Can you work these out from the model? Positions are in its coordinate system, mm. A direction names the side the tool comes from. Coordinates: 2 decimals unless noted, no trailing zeros. Write each loop counter-clockwise with the first axis right and the second up, starting at its lowest first coordinate (ties: lowest second). Pieces come first, ordered by that corner, then holes. Notation, with made-up numbers: (5.25, -40) -> (60.25, -40) arc R18 cw to (60.25, -23) -> close; hole circle Ø3 at (-28, -9). An arc over 180 degrees is marked (long way). Answer as CSV lines item,"result". Start each with the question number.
```python
from build123d import *

# Parameters (mm, degrees)
SKETCH1_R                    = 2.5
BASE_FLANGE1_DEPTH           = 3
EDGE_FLANGE1_STRIP_W         = 13.4732
EDGE_FLANGE1_STRIP_H         = 3
EDGE_FLANGE1_STRIP_CUT_DEPTH = 54
EDGE_FLANGE1_DEPTH           = 54
CUT_EXTRUDE1_START           = 16
CUT_EXTRUDE1_DEPTH           = 22
SKETCH10_R                   = 2.5
CUT_EXTRUDE2_DEPTH           = 10
SKETCH11_W                   = 22
SKETCH11_H                   = 16
SKETCH11_R                   = 2.5
BOSS_EXTRUDE1_DEPTH          = 3


# Read off the part's stored shape, not the designer's step: Cut-Extrude1
# Sheet-metal steps are written as plain solids
with BuildPart() as part:
    # Sketch1 → Base-Flange1 (new body)
    with BuildSketch(Plane(origin=(0, 0, 0), x_dir=(1, 0, 0), z_dir=(0, 1, 0))):
        with BuildLine():
            Line((0, 0), (54, 0))
            Line((54, 0), (54, 11))
            ThreePointArc((54, 11), (52.535533906, 14.535533906), (49, 16))
            Line((49, 16), (5, 16))
            ThreePointArc((5, 16), (1.464466094, 14.535533906), (0, 11))
            Line((0, 11), (0, 0))
        make_face()
        with Locations(Location((8, 8, 0), (0, 0, 270))):
            Circle(SKETCH1_R, mode=Mode.SUBTRACT)
        with Locations(Location((46, 8, 0), (0, 0, 90))):
            Circle(SKETCH1_R, mode=Mode.SUBTRACT)
    extrude(amount=-BASE_FLANGE1_DEPTH)

    # Edge-Flange1 strip (across the edge) → Edge-Flange1 strip cut (cut)
    with BuildSketch(Plane(origin=(0, 0, 0), x_dir=(0, 0, -1), z_dir=(1, 0, 0))):
        with Locations((-6, -1.5)):
            Rectangle(EDGE_FLANGE1_STRIP_W, EDGE_FLANGE1_STRIP_H)
    extrude(amount=EDGE_FLANGE1_STRIP_CUT_DEPTH, mode=Mode.SUBTRACT)

    # Edge-Flange1 section (across the edge) → Edge-Flange1 (add)
    with BuildSketch(Plane(origin=(0, 0, 0), x_dir=(0, 0, -1), z_dir=(1, 0, 0))):
        with BuildLine():
            Line((-3, 0.7366), (-3, 24))
            Line((-3, 24), (0, 24))
            Line((0, 24), (0, 0.7366))
            ThreePointArc((0, 0.7366), (0.215745145, 0.215745145), (0.7366, 0))
            Line((0.7366, 0), (0.7366, -3))
            ThreePointArc((0.7366, -3), (-1.905575199, -1.905575199), (-3, 0.7366))
        make_face()
    extrude(amount=EDGE_FLANGE1_DEPTH)

    # Cut-Extrude1 outline → Cut-Extrude1 (cut)
    with BuildSketch(Plane.YZ.offset(CUT_EXTRUDE1_START)):
        with BuildLine():
            Line((-2.926677222, 0), (0.014454199, -0.591393245))
            ThreePointArc((0.014454199, -0.591393245), (0.269898669, -0.166714548), (0.7366, 0))
            Line((0.7366, 0), (24, 0))
            Line((24, 0), (24, 3))
            Line((24, 3), (0.7366, 3))
            ThreePointArc((0.7366, 3), (-1.630867001, 2.154295979), (-2.926677222, 0))
        make_face()
    extrude(amount=CUT_EXTRUDE1_DEPTH, mode=Mode.SUBTRACT)

    # Sketch10 → Cut-Extrude2 (cut)
    with BuildSketch(Plane.XY.offset(3)):
        with BuildLine():
            ThreePointArc((46, 24), (51.656854249, 21.656854249), (54, 16))
            Line((54, 16), (54, 24))
            Line((54, 24), (46, 24))
        make_face()
        with Locations((46, 16)):
            Circle(SKETCH10_R)
        with Locations((8, 16)):
            Circle(SKETCH10_R)
        with BuildLine():
            ThreePointArc((0, 16), (2.343145751, 21.656854249), (8, 24))
            Line((8, 24), (0, 24))
            Line((0, 24), (0, 16))
        make_face()
    extrude(amount=-CUT_EXTRUDE2_DEPTH, mode=Mode.SUBTRACT)

    # Sketch11 → Boss-Extrude1 (add)
    with BuildSketch(Plane.XY.offset(3)):
        with Locations((27, 16)):
            Rectangle(SKETCH11_W, SKETCH11_H)
        with Locations((27, 16)):
            Circle(SKETCH11_R, mode=Mode.SUBTRACT)
    extrude(amount=-BOSS_EXTRUDE1_DEPTH)


solid = part.part
```
Q1. Which directions (+Z, -Z, +X, -X, +Y, -Y) give clear straight access to the entire face, cutting with the end or side of a thin tool? Please do faces 1 (the face through (53, -1, -14)), 2 (the face through (27, 13, 0)).
Q2. I need wall thicknesses on L1, parallel to X at y = -1.6, z = -8; L2, parallel to Y at x = 27, z = 2.2; L3, parallel to Z at x = 14.5, y = 3.75. Which ranges of each line are inside material? Lowest first, please.
Q3. Imagine slicing it at B-B (z = -8). Write out the boundary of the cut face in (x, y).
Q4. Imagine slicing it at C-C (z = -14). Write out the boundary of the cut face in (x, y), then the cut area to 3 significant figures.
Q5. For pin 1 (10 mm diameter, centred on x = 44, z = -2.5, fed in from +Y); pin 2 (0.9 mm diameter, centred on x = 26.5, z = 1.5, fed in from -Y); pin 3 (6 mm diameter, centred on x = 8, z = -8, fed in from +Y), each with a flat end and sliding along its axis, tell me the tip position at first contact or that it passes through.
Q6. If we mould it in two halves opening along X, with no side actions, what happens to faces 3 (the face through (54, 4, 1)), 4 (the face through (10.31, 15.04, 1.52)), 5 (the face through (16, 2, 1)), 6 (the face through (27, 0, -8))? For each: released by +X, released by -X, zero draft, split by the parting line, or undercut.
Q7. Imagine slicing it at A-A (x = 23). Write out the boundary of the cut face in (y, z), then the cut area to 3 significant figures.
Q8. Imagine slicing it at D-D (y = 10.5). Write out the boundary of the cut face in (x, z).
Entries:
1,face 1,"-Z, +X, +Y, -Y"
1,face 2,"-Z, +X, -X, +Y"
2,L1,"0 to 5.5, 10.5 to 43.5, 48.5 to 54"
2,L2,"8 to 13.5, 18.5 to 24"
2,L3,"0 to 3"
3,outline,"(0, -3) -> (5.5, -3) -> (5.5, 0) -> (0, 0) -> close; (10.5, -3) -> (43.5, -3) -> (43.5, 0) -> (10.5, 0) -> close; (48.5, -3) -> (54, -3) -> (54, 0) -> (48.5, 0) -> close"
4,outline,"(1, -3) -> (53, -3) -> (53, 0) -> (1, 0) -> close"
4,area,"156 mm2"
5,pin 1,"y = 24"
5,pin 2,"y = 8"
5,pin 3,"y = 0"
6,face 3,"released by +X"
6,face 4,"undercut"
6,face 5,"undercut"
6,face 6,"zero draft"
7,outline,"(-3, -16) -> (0, -16) -> (0, -0.74) arc R0.74 cw to (0.01, -0.59) -> (-2.93, 0) arc R3.74 ccw to (-3, -0.74) -> close; (8, 0) -> (24, 0) -> (24, 3) -> (8, 3) -> close"
7,area,"95.1 mm2"
8,outline,"(0, 0) -> (54, 0) -> (54, 3) -> (0, 3) -> close"
